Verification items for the finished model (mm, model axes). Round coordinates to 2 decimals unless told otherwise and drop trailing zeros. Write each loop counter-clockwise with the first axis right and the second up, starting at its lowest first coordinate (ties: lowest second). Pieces come first, ordered by that corner, then holes. Notation, with made-up numbers: M -14,34.5 L -7,34.5 A30 ccw -7,58.5 Z; hole C 25.5,-21 d5. An arc over 180 degrees is marked long. One line per question, with ' | ' between items.
Solid Edge part; units mm, degrees
sketch "Sketch1" plane through (0, 0, 0) normal (0, 0, 1) x (1, 0, 0)
  line L0 (1.5, 8) -> (-1.5, 8)
  line L1 (-1.5, 8) -> (-1.5, 7)
  line L2 (-1.5, 7) -> (1.5, 7)
  line L3 (1.5, 7) -> (1.5, 8)
  circle A0 centre (0, 0) radius 7.5
  dimension "D1" = 1.5
  dimension "D2" = 1.5
extrude "Protrusion1" add sketch "Sketch1" along normal blind 30
sketch "Sketch2" plane through (0, 0, 30) normal (0, 0, 1) x (0, 1, 0)
  circle A0 centre (0, 0) radius 9
  circle A1 centre (0, 0) radius 7.5
extrude "ExtrudedCutout_3" cut sketch "Sketch2" against normal blind 5
sketch "Sketch3" plane through (0, -0.5, 30) normal (0, 0, 1) x (0, 1, 0)
  circle A0 centre (0.5, 0) radius 5
extrude "Cutout1" cut sketch "Sketch3" against normal up to next
extrude "ExtrudedCutout_7" [suppressed]
properties material "Stainless steel"
1. Section check A-A, the plane y = 0. Record the cut outline in (x, z), then the cut area to 3 significant figures.
Results:
outline: M -7.5,0 L -5,0 L -5,30 L -7.5,30 Z; M 5,0 L 7.5,0 L 7.5,30 L 5,30 Z | area: 150 mm2
2. Section check D-D, the plane x = -6.25. Record the cut outline in (y, z), then the cut area to 3 significant figures.
Results:
outline: M -4.15,0 L 4.15,0 L 4.15,30 L -4.15,30 Z | area: 249 mm2
3. Section check B-B, the plane x = 4.25. Record the cut outline in (y, z).
Results:
outline: M -6.18,0 L -2.63,0 L -2.63,30 L -6.18,30 Z; M 2.63,0 L 6.18,0 L 6.18,30 L 2.63,30 Z
4. Go/stop test with flat-tipped pins: P1, Ø3, axis at y = 3.5, z = 13, coming from the -X side; P2, Ø0.5, axis at y = 8, z = 17, coming from the -X side; P3, Ø6, axis at x = 0, y = 0, coming from the +Z side; P4, Ø1.5, axis at x = 5, z = 26.5, coming from the +Y side. Record where each tip stops, or that it passes through.
Results:
P1: stops at x = -7.23 | P2: stops at x = -1.5 | P3: passes through | P4: stops at y = 6.18
5. Thickness scan on line 1 (Y direction, x = 0, z = 19.5); line 2 (X direction, y = 0, z = 20.75); line 3 (X direction, y = -1, z = 3.5). Record the ranges inside material, lowest first.
Results:
line 1: y = -7.5 to -5, 5 to 8 | line 2: x = -7.5 to -5, 5 to 7.5 | line 3: x = -7.43 to -4.9, 4.9 to 7.43
6. Mould release check, pull along Y, two halves, no side actions. Record for faces 1 (the face through (4.88, -1.08, 15.21)), 2 (the face through (5, -2, 30)), 3 (the face through (0, 8, 12)): pulls with the +Y half, pulls with the -Y half, needs draft (parallel to the pull), parting line crosses it, or undercut.
Results:
face 1: undercut | face 2: needs draft | face 3: pulls with the +Y half
7. Section check C-C, the plane z = 6.25. Record the cut outline in (x, y), then the cut area to 3 significant figures.
Results:
outline: M -1.5,7.35 A7.5 ccw long 1.5,7.35 L 1.5,8 L -1.5,8 Z; hole C 0,0 d10 | area: 99.8 mm2
